from build123d import *

# Parameters (mm, degrees)
SKETCH1_W           = 61.9125
SKETCH1_H           = 22.225
BOSS_EXTRUDE1_DEPTH = 34.925
SKETCH2_W           = 22.225
SKETCH2_H           = 28.575
BOSS_EXTRUDE2_DEPTH = 28.575
SKETCH3_W           = 28.575
SKETCH3_H           = 22.225
BOSS_EXTRUDE3_DEPTH = 28.575
SKETCH5_R           = 6.35
BOSS_EXTRUDE5_DEPTH = 6.35
FILLET1_R           = 3.81
SKETCH6_R           = 9.525
BOSS_EXTRUDE6_DEPTH = 19.05


with BuildPart() as part:
    # Sketch1 → Boss-Extrude1 (new body)
    with BuildSketch(Plane(origin=(0, 0, 0), x_dir=(1, 0, 0), z_dir=(0, 1, 0))):
        with Locations((30.95625, 11.1125)):
            Rectangle(SKETCH1_W, SKETCH1_H)
    extrude(amount=BOSS_EXTRUDE1_DEPTH)

    # Sketch2 → Boss-Extrude2 (add)
    with BuildSketch(Plane.ZY):
        with Locations((-11.1125, 20.6375)):
            Rectangle(SKETCH2_W, SKETCH2_H)
    extrude(amount=BOSS_EXTRUDE2_DEPTH)

    # Sketch3 → Boss-Extrude3 (add)
    with BuildSketch(Plane(origin=(0, 34.925, 0), x_dir=(1, 0, 0), z_dir=(0, 1, 0))):
        with Locations((-14.2875, 11.1125)):
            Rectangle(SKETCH3_W, SKETCH3_H)
    extrude(amount=BOSS_EXTRUDE3_DEPTH)

    # Sketch5 → Boss-Extrude5 (add)
    with BuildSketch(Plane.ZY.offset(28.575)):
        with Locations((-11.1125, 15.875)):
            Circle(SKETCH5_R)
    extrude(amount=BOSS_EXTRUDE5_DEPTH)

    # Fillet1
    fillet1_edges = [part.edges().sort_by_distance(p)[0] for p in [
        (-14.2875, 6.35, -22.225),
        (-14.2875, 6.35, 0),
    ]]
    fillet(fillet1_edges, radius=FILLET1_R)

    # Sketch6 → Boss-Extrude6 (add)
    with BuildSketch(Plane.ZY.offset(28.575)):
        with Locations(Location((-11.1125, 53.975, 0), (0, 0, 90))):
            Circle(SKETCH6_R)
    extrude(amount=BOSS_EXTRUDE6_DEPTH)


solid = part.part
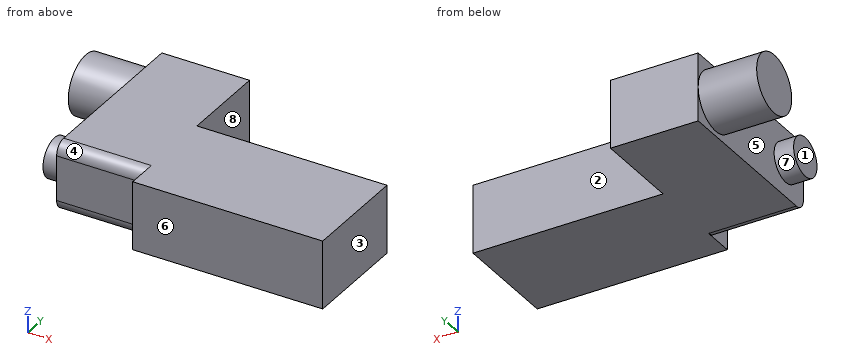
Can you work these out from the model? Positions are in its coordinate system, mm. Face numbers are marked on the shaded views. A direction names the side the tool comes from. Coordinates: 2 decimals unless noted, no trailing zeros. Loops run counter-clockwise (first coordinate to the right, second up) from the corner with the lowest first, then second, coordinate; pieces in that order, holes last. Notation, with made-up numbers: (22.25, 0) - (42.25, 0) arc R29 cw to (42.25, 27) - close; hole circle Ø3 at (50, 65). An arc over 180 degrees is marked (long way). Answer as a JSON object with one key per item and string values. Group by question number.
Item 1: If I drill on L1, parallel to X at y = 55, z = -13.5 (3 decimals); L2, parallel to Y at x = 40.5, z = -14.75 (3 decimals); L3, parallel to X at y = 27.5, z = -8 (1 decimal), over which ranges is the centre line in solid material (lowest first)? Write a range as from..to.
Item 2: For pin 1 (1 mm diameter, centred on y = 13, z = -5, fed in from -X) (3 decimals); pin 2 (11 mm diameter, centred on y = 4, z = -8.5, fed in from -X) (3 decimals); pin 3 (6 mm diameter, centred on x = -11.5, z = -16.5, fed in from -Y), each with a flat end and sliding along its axis, tell me the tip position at first contact or that it passes through.
Item 3: On a 3-axis mill with a long thin cutter (end or side, diameter ignored), from which of +Z, -Z, +X, -X, +Y, -Y can I reach the whole of each face in a straight line? I mean the marked faces 1, 2, 3, 4 and 5. Say none if no direction works.
Item 4: If we section it at C-C (y = 52): List the corners of the cut face in (x, z) for me (1 decimal), plus the area to 3 significant figures.
Item 5: If we mould it in two halves opening along Y, with no side actions, what happens to the marked faces 6, 7 and 8? For each: released by +Y, released by -Y, zero draft, split by the parting line, or undercut.
Item 6: If we section it at A-A (x = -6): List the corners of the cut face in (y, z) for me (3 decimals), plus the area to 3 significant figures.
Returned:
{
 "1": {"L1": "x = -47.625..0", "L2": "y = 0..34.925", "L3": "x = -28.6..61.9"},
 "2": {"pin 1": "stops at x = -34.925", "pin 2": "stops at x = -28.575", "pin 3": "stops at y = 6.35"},
 "3": {"face 1": "+Z, -Z, -X, -Y", "face 2": "+Z, -Z, +X, +Y", "face 3": "+Z, -Z, +X, +Y, -Y", "face 4": "+Z, -X, -Y", "face 5": "-X"},
 "4": {"outline": "(-47.6, -20.4) - (-28.6, -20.4) - (-28.6, -22.2) - (0, -22.2) - (0, 0) - (-28.6, 0) - (-28.6, -1.8) - (-47.6, -1.8) - close", "area": "990 mm²"},
 "5": {"face 6": "released by -Y", "face 7": "undercut", "face 8": "zero draft"},
 "6": {"outline": "(6.35, -18.415) arc R3.81 ccw to (10.16, -22.225) - (63.5, -22.225) - (63.5, 0) - (10.16, 0) arc R3.81 ccw to (6.35, -3.81) - close", "area": "1,260 mm²"}
}
